Input: part model. Units: mm. Frame: model coordinates. A direction names the side the tool comes from. Give positions to 0.01 mm unless a question says otherwise; leave off trailing zeros. Loops run counter-clockwise (first coordinate to the right, second up) from the corner with the lowest first, then second, coordinate; pieces in that order, holes last. Notation, with made-up numbers: (60, 68) -> (75, 68) arc R26 ccw to (75, 103) -> close; hole circle Ø4 at (-1, 35). An arc over 180 degrees is marked (long way). Use CSV: the item, a comma, the result in double quotes.
```python
from build123d import *

# Parameters (mm, degrees)
SKETCH2_R               = 2.4384
BOSS_EXTRUDE1_DEPTH     = 10.5664
CUT_EXTRUDE2_DEPTH      = 97.46498413
CUT_EXTRUDE3_DEPTH      = 3.302
CUT_EXTRUDE3_DEPTH_BACK = 3.302
SKETCH4_R               = 10.31875
FILLET10_R              = 1.27


with BuildPart() as part:
    # Sketch2 → Boss-Extrude1 (new body)
    with BuildSketch(Plane(origin=(0, 0, 0), x_dir=(0, 0, -1), z_dir=(1, 0, 0))):
        with BuildLine():
            Line((-1.887455194, -10.8204), (72.898, -10.8204))
            ThreePointArc((72.898, -10.8204), (75.14306403, -11.75033597), (76.073, -13.9954))
            Line((76.073, -13.9954), (76.073, -18.7579))
            ThreePointArc((76.073, -18.7579), (84.074, -26.7589), (92.075, -18.7579))
            Line((92.075, -18.7579), (92.075, 0))
            Line((92.075, 0), (11.009993871, 0))
            Line((11.009993871, 0), (-14.290030059, 14.938561947))
            ThreePointArc((-14.290030059, 14.938561947), (-26.081703159, 12.683140313), (-22.361521098, 1.268643974))
            Line((-22.361521098, 1.268643974), (-1.887455194, -10.8204))
        make_face()
        with Locations((84.074, -18.7579)):
            Circle(SKETCH2_R, mode=Mode.SUBTRACT)
        with Locations((-19.1920645, 8.615108829)):
            Circle(SKETCH2_R, mode=Mode.SUBTRACT)
    extrude(amount=BOSS_EXTRUDE1_DEPTH)

    # Sketch3 → Cut-Extrude2 (cut, through all)
    with BuildSketch(Plane.ZY):
        with BuildLine():
            ThreePointArc((-6.845534188, -7.643088177), (-5.493822647, -7.817545717), (-4.7625, -6.667447152))
            Line((-4.7625, -6.667447152), (-4.7625, -2.71145))
            ThreePointArc((-4.7625, -2.71145), (-5.134474388, -1.813424388), (-6.0325, -1.44145))
            Line((-6.0325, -1.44145), (-10.779696582, -1.44145))
            ThreePointArc((-10.779696582, -1.44145), (-11.973841486, -2.279109915), (-11.59273077, -3.687091025))
            Line((-11.59273077, -3.687091025), (-6.845534188, -7.643088177))
        make_face()
        with BuildLine():
            ThreePointArc((-17.4625, -8.10895), (-17.090525612, -9.006975612), (-16.1925, -9.37895))
            Line((-16.1925, -9.37895), (-11.445303418, -9.37895))
            ThreePointArc((-11.445303418, -9.37895), (-10.251158514, -8.541290085), (-10.63226923, -7.133308975))
            Line((-10.63226923, -7.133308975), (-15.379465812, -3.177311823))
            ThreePointArc((-15.379465812, -3.177311823), (-16.731177353, -3.002854283), (-17.4625, -4.152952848))
            Line((-17.4625, -4.152952848), (-17.4625, -8.10895))
        make_face()
        with BuildLine():
            ThreePointArc((-21.133034188, -7.643088177), (-19.781322647, -7.817545717), (-19.05, -6.667447152))
            Line((-19.05, -6.667447152), (-19.05, -2.71145))
            ThreePointArc((-19.05, -2.71145), (-19.421974388, -1.813424388), (-20.32, -1.44145))
            Line((-20.32, -1.44145), (-25.067196582, -1.44145))
            ThreePointArc((-25.067196582, -1.44145), (-26.261341486, -2.279109915), (-25.88023077, -3.687091025))
            Line((-25.88023077, -3.687091025), (-21.133034188, -7.643088177))
        make_face()
        with BuildLine():
            ThreePointArc((-31.75, -8.10895), (-31.378025612, -9.006975612), (-30.48, -9.37895))
            Line((-30.48, -9.37895), (-25.732803418, -9.37895))
            ThreePointArc((-25.732803418, -9.37895), (-24.538658514, -8.541290085), (-24.91976923, -7.133308975))
            Line((-24.91976923, -7.133308975), (-29.666965812, -3.177311823))
            ThreePointArc((-29.666965812, -3.177311823), (-31.018677353, -3.002854283), (-31.75, -4.152952848))
            Line((-31.75, -4.152952848), (-31.75, -8.10895))
        make_face()
        with BuildLine():
            ThreePointArc((-35.420534188, -7.643088177), (-34.068822647, -7.817545717), (-33.3375, -6.667447152))
            Line((-33.3375, -6.667447152), (-33.3375, -2.71145))
            ThreePointArc((-33.3375, -2.71145), (-33.709474388, -1.813424388), (-34.6075, -1.44145))
            Line((-34.6075, -1.44145), (-39.354696582, -1.44145))
            ThreePointArc((-39.354696582, -1.44145), (-40.548841486, -2.279109915), (-40.16773077, -3.687091025))
            Line((-40.16773077, -3.687091025), (-35.420534188, -7.643088177))
        make_face()
        with BuildLine():
            ThreePointArc((-46.0375, -8.10895), (-45.665525612, -9.006975612), (-44.7675, -9.37895))
            Line((-44.7675, -9.37895), (-40.020303418, -9.37895))
            ThreePointArc((-40.020303418, -9.37895), (-38.826158514, -8.541290085), (-39.20726923, -7.133308975))
            Line((-39.20726923, -7.133308975), (-43.954465812, -3.177311823))
            ThreePointArc((-43.954465812, -3.177311823), (-45.306177353, -3.002854283), (-46.0375, -4.152952848))
            Line((-46.0375, -4.152952848), (-46.0375, -8.10895))
        make_face()
        with BuildLine():
            ThreePointArc((-49.708034188, -7.643088177), (-48.356322647, -7.817545717), (-47.625, -6.667447152))
            Line((-47.625, -6.667447152), (-47.625, -2.71145))
            ThreePointArc((-47.625, -2.71145), (-47.996974388, -1.813424388), (-48.895, -1.44145))
            Line((-48.895, -1.44145), (-53.642196582, -1.44145))
            ThreePointArc((-53.642196582, -1.44145), (-54.836341486, -2.279109915), (-54.45523077, -3.687091025))
            Line((-54.45523077, -3.687091025), (-49.708034188, -7.643088177))
        make_face()
        with BuildLine():
            ThreePointArc((-60.325, -8.10895), (-59.953025612, -9.006975612), (-59.055, -9.37895))
            Line((-59.055, -9.37895), (-54.307803418, -9.37895))
            ThreePointArc((-54.307803418, -9.37895), (-53.113658514, -8.541290085), (-53.49476923, -7.133308975))
            Line((-53.49476923, -7.133308975), (-58.241965812, -3.177311823))
            ThreePointArc((-58.241965812, -3.177311823), (-59.593677353, -3.002854283), (-60.325, -4.152952848))
            Line((-60.325, -4.152952848), (-60.325, -8.10895))
        make_face()
        with BuildLine():
            ThreePointArc((-82.882803418, -9.37895), (-81.688658514, -8.541290085), (-82.06976923, -7.133308975))
            Line((-82.06976923, -7.133308975), (-86.816965812, -3.177311823))
            ThreePointArc((-86.816965812, -3.177311823), (-88.168677353, -3.002854283), (-88.9, -4.152952848))
            Line((-88.9, -4.152952848), (-88.9, -8.10895))
            ThreePointArc((-88.9, -8.10895), (-88.528025612, -9.006975612), (-87.63, -9.37895))
            Line((-87.63, -9.37895), (-82.882803418, -9.37895))
        make_face()
        with BuildLine():
            ThreePointArc((-78.283034188, -7.643088177), (-76.931322647, -7.817545717), (-76.2, -6.667447152))
            Line((-76.2, -6.667447152), (-76.2, -2.71145))
            ThreePointArc((-76.2, -2.71145), (-76.571974388, -1.813424388), (-77.47, -1.44145))
            Line((-77.47, -1.44145), (-82.217196582, -1.44145))
            ThreePointArc((-82.217196582, -1.44145), (-83.411341486, -2.279109915), (-83.03023077, -3.687091025))
            Line((-83.03023077, -3.687091025), (-78.283034188, -7.643088177))
        make_face()
        with BuildLine():
            ThreePointArc((-74.6125, -8.10895), (-74.240525612, -9.006975612), (-73.3425, -9.37895))
            Line((-73.3425, -9.37895), (-68.595303418, -9.37895))
            ThreePointArc((-68.595303418, -9.37895), (-67.401158514, -8.541290085), (-67.78226923, -7.133308975))
            Line((-67.78226923, -7.133308975), (-72.529465812, -3.177311823))
            ThreePointArc((-72.529465812, -3.177311823), (-73.881177353, -3.002854283), (-74.6125, -4.152952848))
            Line((-74.6125, -4.152952848), (-74.6125, -8.10895))
        make_face()
        with BuildLine():
            ThreePointArc((-63.995534188, -7.643088177), (-62.643822647, -7.817545717), (-61.9125, -6.667447152))
            Line((-61.9125, -6.667447152), (-61.9125, -2.71145))
            ThreePointArc((-61.9125, -2.71145), (-62.284474388, -1.813424388), (-63.1825, -1.44145))
            Line((-63.1825, -1.44145), (-67.929696582, -1.44145))
            ThreePointArc((-67.929696582, -1.44145), (-69.123841486, -2.279109915), (-68.74273077, -3.687091025))
            Line((-68.74273077, -3.687091025), (-63.995534188, -7.643088177))
        make_face()
    extrude(amount=-CUT_EXTRUDE2_DEPTH, mode=Mode.SUBTRACT)

    # Sketch4 → Cut-Extrude3 (cut, two sides: drawn at the far end of the back side and taken through both)
    with BuildSketch(Plane(origin=(5.2832, 0, 0), x_dir=(0, 0, -1), z_dir=(1, 0, 0)).offset(-CUT_EXTRUDE3_DEPTH_BACK)):
        with Locations((-19.1920645, 8.615108829)):
            Circle(SKETCH4_R)
        with Locations((84.074, -18.7579)):
            Circle(SKETCH4_R)
    extrude(amount=CUT_EXTRUDE3_DEPTH + CUT_EXTRUDE3_DEPTH_BACK, mode=Mode.SUBTRACT)

    # Fillet10
    fillet10_edges = [part.edges().sort_by_distance(p)[0] for p in [
        (10.5664, -26.7589, -84.074),
        (0, -11.75033597, -75.14306403),
        (0, -10.8204, -35.505272403),
        (0, -4.775878013, 12.124488146),
        (0, 7.469280973, 1.640018094),
        (0, 0, -51.542496936),
        (10.5664, -9.37895, -92.075),
        (0, -9.37895, -92.075),
        (0, -26.7589, -84.074),
        (0, -16.37665, -76.073),
        (5.2832, -10.8204, 1.887455194),
        (10.5664, 0, -51.542496936),
        (10.5664, 7.469280973, 1.640018094),
        (10.5664, -4.775878013, 12.124488146),
        (10.5664, 12.683140313, 26.081703159),
        (0, 12.683140313, 26.081703159),
        (10.5664, -10.8204, -35.505272403),
        (10.5664, -11.75033597, -75.14306403),
        (10.5664, -16.37665, -76.073),
    ]]
    fillet(fillet10_edges, radius=FILLET10_R)


solid = part.part
```
1) Ray query, line 1 (Y direction, x = 4.5, z = -40); line 2 (Y direction, x = 8.25, z = -72); line 3 (Y direction, x = 9.25, z = -20). Return the intervals inside material, ascending.
From the geometry:
line 1,"y = -10.82 to -9.38, -6.47 to -3.83, -1.62 to 0"
line 2,"y = -10.82 to -9.38, -3.62 to 0"
line 3,"y = -10.82 to -7.9, -1.48 to 0"
2) Section query A-A (z = -56). Return loops of the section in (x, y), then the cut area to 3 significant figures.
From the geometry:
outline,"(0, -9.55) arc R1.27 ccw to (1.27, -10.82) -> (9.3, -10.82) arc R1.27 ccw to (10.57, -9.55) -> (10.57, -9.38) -> (0, -9.38) -> close; (0, -5.05) -> (10.57, -5.05) -> (10.57, -1.27) arc R1.27 ccw to (9.3, 0) -> (1.27, 0) arc R1.27 ccw to (0, -1.27) -> close"
area,"67.2 mm^2"
3) Section query B-B (x = 6.75). Give the number of separate pieces and of enclosed holes in the cut face, then the cut area to 3 significant figures.
From the geometry:
separate pieces,"1"
enclosed holes,"11"
area,"826 mm^2"
4) Reachability of faces 1 (the cylindrical face through (5.21, -8.56, -10.26)), 2 (the cylindrical face through (5.237, -10.104, -78.454)), 3 (the flat face through (5, 0, -52)) from +Z, -Z, +X, -X, +Y, -Y: full face, straight path, thin tool, end or side. Return the list, or none.
From the geometry:
face 1,"+X, -X"
face 2,"-Y"
face 3,"-Z, +X, -X, +Y"
5) Contact query for flat-ended pins moving along their axis: pin 1 (4.5 mm diameter, centred on x = 7.5, y = -6, fed in from +Z); pin 2 (3 mm diameter, centred on x = 6, y = -5.5, fed in from +Z); pin 3 (3 mm diameter, centred on x = 3.5, y = -6.5, fed in from +Z). Output: stop coordinate, or through.
From the geometry:
pin 1,"stops at z = 13.86"
pin 2,"stops at z = 13.44"
pin 3,"stops at z = 11.74"
6) Mould query, pull axis Z, two halves, no side actions, for faces 4 (the cylindrical face through (9.562, 7.131, 21.127)), 5 (the flat face through (0, -2, -28)), 6 (the flat face through (5.227, 5.705, -1.348)). Classes: pulls with the +Z half, pulls with the -Z half, needs draft (parallel to the pull), parting line crosses it, or undercut.
From the geometry:
face 4,"undercut"
face 5,"needs draft"
face 6,"pulls with the -Z half"
